Design review of the part built by this model. Coordinates are the model's own, in mm. A direction names the side the tool comes from. Coordinates: 2 decimals unless noted, no trailing zeros. Order: outer loops, then holes, each group sorted by start corner. A loop starts at its lowest first (then second) coordinate and runs counter-clockwise, first axis right, second up. Notation, with made-up numbers: (64.5, 54.25) -> (114.5, 54.25) arc R8 ccw to (114.5, 59.25) -> close; hole circle Ø11 at (71.25, 18). An arc over 180 degrees is marked (long way). Use a Markdown table: item, result. Add a question column.
Q1. Insertion check: pin 1 (1.5 mm diameter, centred on y = 4, z = 17.5, fed in from +X); pin 2 (1.5 mm diameter, centred on y = -3.5, z = -116.5, fed in from -X); pin 3 (3 mm diameter, centred on x = 1, z = -128.5, fed in from +Y); pin 4 (1 mm diameter, centred on y = 2, z = -92, fed in from -X). Each pin has a flat end and moves straight along its axis. Give the tip position at first contact, or say it passes through.
Q2. Wall thickness on probe 1 along Y at (x, z) = (-0.25, 34.5); probe 2 along Y at (x, z) = (-4.5, 91): over which ranges is each line inside the solid? List them lowest first.
Q3. Add section C-C (z = -154). State the section outline as (x, y) points.
Q4. Machinability: for faces 1 (the face through (-0.867, -3.905, 175.07)), 2 (the face through (-0.867, -3.905, -175.07)), 3 (the face through (0, 0, -180)), which of the approach directions +Z, -Z, +X, -X, +Y, -Y give a long, thin tool a straight path to every point of the face, cutting with its end or side? Answer none if there is none.
from build123d import *

# Parameters (mm, degrees)
SKETCH1_R            = 6
BOSS_EXTRUDE1_DEPTH  = 180
SKETCH2_R            = 6
SKETCH2_R_2          = 4
CUT_EXTRUDE1_DEPTH   = 10
FILLET1_R            = 2
FILLET1_OF_MIRROR1_R = 2


with BuildPart() as part:
    # Sketch1 → Boss-Extrude1 (new, symmetric)
    with BuildSketch(Plane.XY):
        with Locations(Location((0, 0, 0), (0, 0, 180))):
            Circle(SKETCH1_R)
    extrude(amount=BOSS_EXTRUDE1_DEPTH, both=True)

    # Sketch2 → Cut-Extrude1 (cut)
    with BuildSketch(Plane.XY.offset(180)):
        with Locations(Location((0, 0, 0), (0, 0, 180))):
            Circle(SKETCH2_R)
        Circle(SKETCH2_R_2, mode=Mode.SUBTRACT)
    cut_extrude1 = extrude(amount=-CUT_EXTRUDE1_DEPTH, mode=Mode.SUBTRACT)

    # Fillet1
    fillet1_edges = [part.edges().sort_by_distance(p)[0] for p in [
        (6, 0, 170),
    ]]
    fillet(fillet1_edges, radius=FILLET1_R - 0.0001)  # a hair under: the kernel refuses the full size

    # Mirror1: Cut-Extrude1 across plane
    add(cut_extrude1.mirror(Plane.XY), mode=Mode.SUBTRACT)

    # Fillet1 of Mirror1
    fillet1_of_mirror1_edges = [part.edges().sort_by_distance(p)[0] for p in [
        (6, 0, -170),
    ]]
    fillet(fillet1_of_mirror1_edges, radius=FILLET1_OF_MIRROR1_R - 0.0001)  # a hair under: the kernel refuses the full size


solid = part.part
Established:
| question | item | result |
|---|---|---|
| 1 | pin 1 | x = 5.04 |
| 1 | pin 2 | x = -5.33 |
| 1 | pin 3 | y = 6 |
| 1 | pin 4 | x = -5.81 |
| 2 | probe 1 | -5.99 to 5.99 |
| 2 | probe 2 | -3.97 to 3.97 |
| 3 | outline | circle Ø12 at (0, 0) |
| 4 | face 1 | +Z |
| 4 | face 2 | -Z |
| 4 | face 3 | -Z, +X, -X, +Y, -Y |
